```python
from build123d import *

# Parameters (mm, degrees)
F0_R     = 8.875
F1_DEPTH = 8
F2_SIZE  = 1


with BuildPart() as f1:
    # F0 (on Front) → F1 (new body)
    with BuildSketch(Plane.XZ):
        with BuildLine():
            ThreePointArc((0, 10.475), (7.071068, 7.728236), (10.433771, 0.928461))
            Line((10.433771, 0.928461), (9.461263, 22.829172))
            Line((9.461263, 22.829172), (0, 22.409042))
            Line((0, 22.409042), (0.528892, 22.385556))
            Line((0.528892, 22.385556), (0, 10.475))
        make_face()
        Polygon((-0.528892, 22.385556), (0, 10.475), (0.528892, 22.385556), (0, 22.409042), align=None)
        with BuildLine():
            Line((-10.433771, 0.928461), (-10.475, 0))
            ThreePointArc((-10.475, 0), (0, -10.475), (10.475, 0))
            Line((10.475, 0), (10.433771, 0.928461))
            ThreePointArc((10.433771, 0.928461), (7.071068, 7.728236), (0, 10.475))
            ThreePointArc((0, 10.475), (-7.071068, 7.728236), (-10.433771, 0.928461))
        make_face()
        Circle(F0_R, mode=Mode.SUBTRACT)
        with BuildLine():
            Line((-9.461263, 22.829172), (-10.433771, 0.928461))
            ThreePointArc((-10.433771, 0.928461), (-7.071068, 7.728236), (0, 10.475))
            Line((0, 10.475), (-0.528892, 22.385556))
            Line((-0.528892, 22.385556), (0, 22.409042))
            Line((0, 22.409042), (-9.461263, 22.829172))
        make_face()
    extrude(amount=F1_DEPTH)

    # F2
    f2_edges = [f1.edges().sort_by_distance(p)[0] for p in [
        (-8.875, 0, 0),
        (-8.875, -8, 0),
    ]]
    chamfer(f2_edges, length=F2_SIZE)


solid = f1.part
```
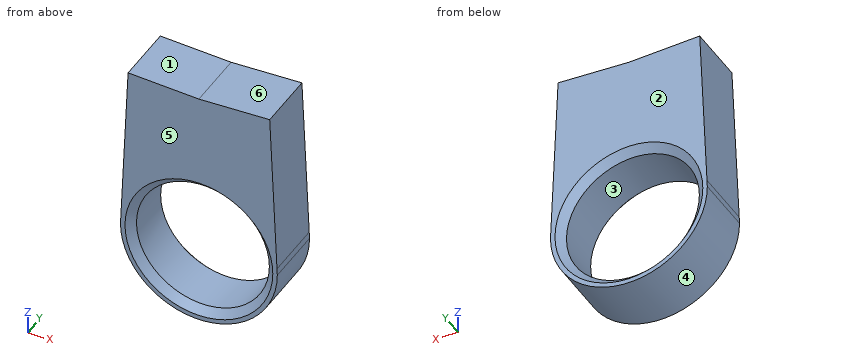
Verification items for the finished model (mm, model axes). Face numbers are marked on the shaded views. A direction names the side the tool comes from. Coordinates: 2 decimals unless noted, no trailing zeros. Loops run counter-clockwise (first coordinate to the right, second up) from the corner with the lowest first, then second, coordinate; pieces in that order, holes last. Notation, with made-up numbers: (75.25, -10.75) - (102.25, -10.75) arc R21 ccw to (102.25, 6.25) - close; hole circle Ø5 at (-6.5, 87.5). An arc over 180 degrees is marked (long way). Put each result on its own line as item: value.
Item 1: Section check C-C (z = 17.5). Enter the section's corners in (x, y).
Conclusion:
outline: (-9.7, -8) - (9.7, -8) - (9.7, 0) - (-9.7, 0) - close
Item 2: Draft check along Z on the marked faces 1, 2, 3 and 4. Enter one of: pulls with the +Z half, pulls with the -Z half, needs draft (parallel to the pull), parting line crosses it, or undercut.
Conclusion:
face 1: pulls with the +Z half
face 2: needs draft
face 3: undercut
face 4: pulls with the -Z half
Item 3: Scan lines: line 1 along Z through (x, y) = (0, -4.45) (3 decimals); line 2 along Z through (x, y) = (-6, -6.5); line 3 along X through (y, z) = (-7.25, -8). Record each from-to range of solid material in increasing order.
Conclusion:
line 1: z = -10.475 to -8.875, 8.875 to 22.409
line 2: z = -8.59 to -6.54, 6.54 to 22.68
line 3: x = -6.76 to -4.39, 4.39 to 6.76
Item 4: Gauge pin test, flat ends, axial feed: pin 1 Ø1 at (y, z) = (-6, 18) entering from -X; pin 2 Ø4 at (x, z) = (-6, -2.5) entering from +Y; pin 3 Ø2 at (y, z) = (-3, 6) entering from +X. Record the tip position at first contact, or that the pin passes through.
Conclusion:
pin 1: stops at x = -9.7
pin 2: passes through
pin 3: stops at x = 10.25
Item 5: Section check A-A (y = -2). Enter the section's corners in (x, z) (3 decimals).
Conclusion:
outline: (-10.475, 0) arc R10.475 ccw to (10.475, 0) - (10.434, 0.928) - (9.461, 22.829) - (0, 22.409) - (-9.461, 22.829) - (-10.434, 0.928) - close; hole circle Ø17.75 at (0, 0)
Item 6: Set-up check for the marked faces 5 and 6: record each of +Z, -Z, +X, -X, +Y, -Y from which the full face is reachable in a straight line by a thin tool's end or side.
Conclusion:
face 5: +Z, -Z, +X, -X, -Y
face 6: +Z, +Y, -Y
Item 7: Section check B-B (z = 11.5). Enter the section's corners in (x, y), then the cut area to 3 significant figures.
Conclusion:
outline: (-9.96, -8) - (9.96, -8) - (9.96, 0) - (-9.96, 0) - close
area: 159 mm2
